Part model, mm, in its own coordinate system. A direction names the side the tool comes from. Round coordinates to 2 decimals unless told otherwise and drop trailing zeros. Loops run counter-clockwise (first coordinate to the right, second up) from the corner with the lowest first, then second, coordinate; pieces in that order, holes last. Notation, with made-up numbers: M 78,-39.5 L 129,-39.5 A9 ccw 129,-25.5 Z; hole C 87.25,-20 d2. An arc over 180 degrees is marked long. Put each result on its own line as item: value. Start each with the question number.
1) Slice it at D-D on x = 0.6. Give the cut face in (y, z).
2) Drop a flat-ended pin along its axis: pin 1 Ø3 at (x, z) = (2, -4.5) entering from -Y. Give the stop position or say it passes through.
3) Probe line 1 along Z through (x, y) = (1.8, -1.25); line 2 along X through (y, z) = (0.75, -6); line 3 along Z through (x, y) = (2.15, 1.5). List the from-to ranges inside material, lowest first.
4) Slice it at B-B on x = 2.3. Give the cut face in (y, z), then the cut area to 3 significant figures.
5) Pull direction X, two halves, no side cores. Call faces 1 (the flat face through (3, -3, -10.5)), 2 (the flat face through (5.8, 0.4, -5.2)), 3 (the flat face through (3.9, 1, -5)), 4 (the flat face through (0, 0.4, -5.2)): +X half, -X half, draft (parallel to the pull), parting line (faces both ways), or undercut.
6) Which spindle directions (+Z, -Z, +X, -X, +Y, -Y) get a long thin tool onto all of the face, cutting with end or side? Do faces 5 (the flat face through (3, -8, -10)), 6 (the flat face through (1.6, 0, -5.3)), 7 (the flat face through (3, 1, -3)). Say none if no direction does.
7) Slice it at C-C on y = -6.5. Give the cut face in (x, z), then the cut area to 3 significant figures.
8) Slice it at A-A on z = -3.25. Give the cut face in (x, y), then the cut area to 3 significant figures.
```python
from build123d import *

# Parameters (mm, degrees)
CROQUIS1_W              = 5.8
CROQUIS1_H              = 10.5
CROQUIS1_W_2            = 2
CROQUIS1_H_2            = 4.5
SALIENTE_EXTRUIR1_DEPTH = 2
CROQUIS2_W              = 5.8
CROQUIS2_H              = 1.2
SALIENTE_EXTRUIR2_DEPTH = 8


with BuildPart() as part:
    # Croquis1 → Saliente-Extruir1 (new body)
    with BuildSketch(Plane(origin=(0, 0, 0), x_dir=(1, 0, 0), z_dir=(0, 1, 0))):
        with Locations((2.9, 5.25)):
            Rectangle(CROQUIS1_W, CROQUIS1_H)
        with Locations((2.9, 5.25)):
            Rectangle(CROQUIS1_W_2, CROQUIS1_H_2, mode=Mode.SUBTRACT)
    extrude(amount=SALIENTE_EXTRUIR1_DEPTH)

    # Croquis2 → Saliente-Extruir2 (add)
    with BuildSketch(Plane(origin=(0, 0, 0), x_dir=(-1, 0, 0), z_dir=(0, -1, 0))):
        with Locations((-2.9, 9.9)):
            Rectangle(CROQUIS2_W, CROQUIS2_H)
        with Locations((-2.9, 0.6)):
            Rectangle(CROQUIS2_W, CROQUIS2_H)
    extrude(amount=SALIENTE_EXTRUIR2_DEPTH)


solid = part.part
```
Recorded:
1. outline: M -8,-10.5 L 2,-10.5 L 2,0 L -8,0 L -8,-1.2 L 0,-1.2 L 0,-9.3 L -8,-9.3 Z
2. pin 1: stops at y = 0
3. line 1: z = -10.5 to -9.3, -1.2 to 0
3. line 2: x = 0 to 1.9, 3.9 to 5.8
3. line 3: z = -10.5 to -7.5, -3 to 0
4. outline: M -8,-10.5 L 2,-10.5 L 2,-7.5 L 0,-7.5 L 0,-9.3 L -8,-9.3 Z; M -8,-1.2 L 0,-1.2 L 0,-3 L 2,-3 L 2,0 L -8,0 Z
4. area: 31.2 mm2
5. face 1: draft
5. face 2: +X half
5. face 3: undercut
5. face 4: -X half
6. face 5: +Z, -Z, +X, -X, -Y
6. face 6: +X, -X, -Y
6. face 7: +Y, -Y
7. outline: M 0,-10.5 L 5.8,-10.5 L 5.8,-9.3 L 0,-9.3 Z; M 0,-1.2 L 5.8,-1.2 L 5.8,0 L 0,0 Z
7. area: 13.9 mm2
8. outline: M 0,0 L 1.9,0 L 1.9,2 L 0,2 Z; M 3.9,0 L 5.8,0 L 5.8,2 L 3.9,2 Z
8. area: 7.60 mm2
